```python
from build123d import *

# Parameters (mm, degrees)
F1_DEPTH = 25


with BuildPart() as f1:
    # F0 (on Front) → F1 (new body)
    with BuildSketch(Plane.XZ):
        with BuildLine():
            Line((223.026821, 17.026341), (155.026801, 17.026341))
            Line((155.026801, 17.026341), (155.026801, 13.526341))
            Line((155.026801, 13.526341), (221.246859, 13.526341))
            ThreePointArc((221.246859, 13.526341), (228.554933, 11.523823), (233.821421, 6.07569))
            ThreePointArc((233.821421, 6.07569), (240.58999, -0.926332), (249.982439, -3.5))
            Line((249.982439, -3.5), (310.053602, -3.5))
            Line((310.053602, -3.5), (310.053602, 0))
            Line((310.053602, 0), (249.982439, 0))
            ThreePointArc((249.982439, 0), (242.011783, 2.306512), (236.50463, 8.513171))
            ThreePointArc((236.50463, 8.513171), (230.997477, 14.71983), (223.026821, 17.026341))
        make_face()
        with BuildLine():
            Line((60.071163, 0), (0, 0))
            Line((0, 0), (0, -3.5))
            Line((0, -3.5), (60.071163, -3.5))
            ThreePointArc((60.071163, -3.5), (69.463611, -0.926332), (76.232181, 6.07569))
            ThreePointArc((76.232181, 6.07569), (81.498668, 11.523823), (88.806743, 13.526341))
            Line((88.806743, 13.526341), (155.026801, 13.526341))
            Line((155.026801, 13.526341), (155.026801, 17.026341))
            Line((155.026801, 17.026341), (87.02678, 17.026341))
            ThreePointArc((87.02678, 17.026341), (79.056125, 14.71983), (73.548972, 8.513171))
            ThreePointArc((73.548972, 8.513171), (68.041819, 2.306512), (60.071163, 0))
        make_face()
    extrude(amount=F1_DEPTH)


solid = f1.part
```
For this review, take the finished solid that the model builds, in its own axes (mm). A direction names the side the tool comes from. Coordinates: 2 decimals unless noted, no trailing zeros. Loops run counter-clockwise (first coordinate to the right, second up) from the corner with the lowest first, then second, coordinate; pieces in that order, holes last. Notation, with made-up numbers: (1.5, 47) - (47.5, 47) arc R22 cw to (47.5, 53) - close; hole circle Ø11 at (58, 58). An arc over 180 degrees is marked (long way). Use one line per item in the form item = value. Start each with the question number.
1) To check wall thickness, follow probe 1 along Z at (x, y) = (50, -9.5); probe 2 along Z at (x, y) = (102, -10.75); probe 3 along X at (y, z) = (-17.5, 5.5). State the ranges of each line that lie inside material, in increasing order. Write a range as from..to.
2) Take a section at C-C (x = 190.5). State the section outline as (y, z) points.
3) Take a section at B-B (y = -5.75). State the section outline as (x, z) points, plus the area to 3 significant figures.
4) For faces 1 (the face through (154, 0, 14)), 2 (the face through (30, -12, 0)), 3 (the face through (280, -12, 0)), 4 (the face through (228.46, -12.32, 11.58)), list the 3-axis set-ups (+Z, -Z, +X, -X, +Y, -Y) from which the entire face can be reached by the end or side of a thin tool; tool diameter is ignored.
5) Draft analysis for pull direction X (two halves, no side actions). For faces 5 (the face through (69.34, -12.32, -1)), 6 (the face through (156, -12, 17.026)), state which applies: released by +X, released by -X, zero draft, split by the parting line, or undercut.
6) For pin 1 (1.5 mm diameter, centred on x = 154, y = -15.5, fed in from -Z); pin 2 (1 mm diameter, centred on x = 249, y = -11, fed in from -Z); pin 3 (1 mm diameter, centred on y = -18.5, z = 5.5, fed in from -X); pin 4 (10 mm diameter, centred on x = 33.5, z = 2.5, fed in from -Y), all flat-tipped, find the tip position at first contact; note any pin that passes through.
7) Take a section at D-D (x = 246). State the section outline as (y, z) points.
8) Take a section at A-A (z = 3.5). State the section outline as (x, y) points.
From the geometry:
q1.probe_1 = -3.5..0
q1.probe_2 = 13.53..17.03
q1.probe_3 = 71.64..75.9, 234.15..238.41
q2.outline = (-25, 13.53) - (0, 13.53) - (0, 17.03) - (-25, 17.03) - close
q3.outline = (0, -3.5) - (60.07, -3.5) arc R18.43 ccw to (76.23, 6.08) arc R14.34 cw to (88.81, 13.53) - (221.25, 13.53) arc R14.34 cw to (233.82, 6.08) arc R18.43 ccw to (249.98, -3.5) - (310.05, -3.5) - (310.05, 0) - (249.98, 0) arc R14.93 cw to (236.5, 8.51) arc R14.93 ccw to (223.03, 17.03) - (87.03, 17.03) arc R14.93 ccw to (73.55, 8.51) arc R14.93 cw to (60.07, 0) - (0, 0) - close
q3.area = 1,140 mm2
q4.face_1 = +Z, -Z, +X, -X, +Y
q4.face_2 = +Z, -X, +Y, -Y
q4.face_3 = +Z, +X, +Y, -Y
q4.face_4 = -Z, +Y, -Y
q5.face_5 = undercut
q5.face_6 = zero draft
q6.pin_1 = 13.53
q6.pin_2 = -3.49
q6.pin_3 = 71.22
q6.pin_4 = -25
q7.outline = (-25, -3.06) - (0, -3.06) - (0, 0.54) - (-25, 0.54) - close
q8.outline = (69.67, -25) - (74.53, -25) - (74.53, 0) - (69.67, 0) - close; (235.53, -25) - (240.38, -25) - (240.38, 0) - (235.53, 0) - close
